```python
from build123d import *

# Parameters (mm, degrees)
F0_R     = 35
F1_DEPTH = 3
F2_R     = 2.75
F3_DEPTH = 3
F4_R     = 26
F5_DEPTH = 3.1
F6_R     = 15
F7_DEPTH = 6.1
F8_SIZE  = 1


with BuildPart() as f1:
    # F0 (on Front) → F1 (new body)
    with BuildSketch(Plane.XZ):
        Circle(F0_R)
    extrude(amount=F1_DEPTH)

    # F2 (on face) → F3 (cut, through all)
    with BuildSketch(Plane.XZ.offset(3)):
        with Locations((30, 0)):
            Circle(F2_R)
        with Locations((0, 30)):
            Circle(F2_R)
        with Locations((-30, 0)):
            Circle(F2_R)
        with Locations((0, -30)):
            Circle(F2_R)
    extrude(amount=-F3_DEPTH, mode=Mode.SUBTRACT)

    # F4 (on face) → F5 (join)
    with BuildSketch(Plane.XZ.offset(3)):
        Circle(F4_R)
    extrude(amount=F5_DEPTH)

    # F6 (on face) → F7 (cut, through all)
    with BuildSketch(Plane.XZ.offset(6.1)):
        Circle(F6_R)
    extrude(amount=-F7_DEPTH, mode=Mode.SUBTRACT)

    # F8
    f8_edges = [f1.edges().sort_by_distance(p)[0] for p in [
        (-26, -6.1, 0),
    ]]
    chamfer(f8_edges, length=F8_SIZE)


solid = f1.part
```
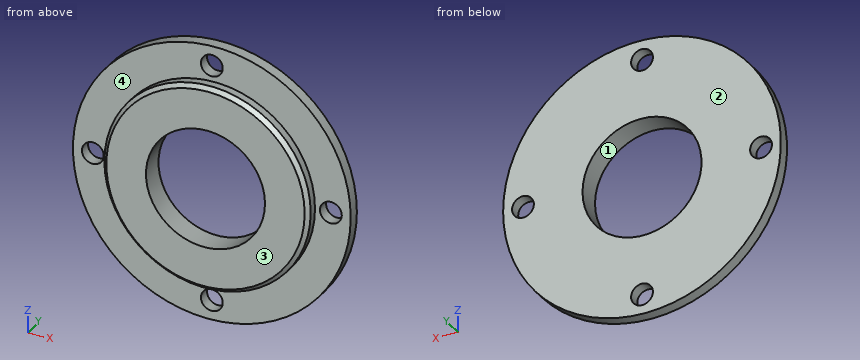
Verification items for the finished model (mm, model axes). Face numbers are marked on the shaded views. A direction names the side the tool comes from. Coordinates: 2 decimals unless noted, no trailing zeros. Loops run counter-clockwise (first coordinate to the right, second up) from the corner with the lowest first, then second, coordinate; pieces in that order, holes last. Notation, with made-up numbers: (69.25, 53.5) -> (107.25, 53.5) arc R13 ccw to (107.25, 63.5) -> close; hole circle Ø6 at (48, 47.25). An arc over 180 degrees is marked (long way). Put each result on its own line as item: value.
1. Thickness scan on line 1 (Z direction, x = 0, y = -2.25); line 2 (Z direction, x = 0, y = -4); line 3 (Z direction, x = -30, y = -1.7). Record the ranges inside material, lowest first.
Result set:
line 1: z = -35 to -32.75, -27.25 to -15, 15 to 27.25, 32.75 to 35
line 2: z = -26 to -15, 15 to 26
line 3: z = -18.03 to -2.75, 2.75 to 18.03
2. Tool access check on the marked faces 3 and 4. Record the directions out of +Z, -Z, +X, -X, +Y, -Y that give a thin tool (end or side, any length) a straight path to the whole face; none if there is none.
Result set:
face 3: +Z, -Z, +X, -X, -Y
face 4: -Y
3. Section check C-C, the plane y = -2. Record the boundary of the cut face in (x, z).
Result set:
outline: circle Ø70 at (0, 0); hole circle Ø5.5 at (-30, 0); hole circle Ø30 at (0, 0); hole circle Ø5.5 at (0, -30); hole circle Ø5.5 at (0, 30); hole circle Ø5.5 at (30, 0)
4. Section check A-A, the plane z = 0. Record the boundary of the cut face in (x, y).
Result set:
outline: (-35, -3) -> (-32.75, -3) -> (-32.75, 0) -> (-35, 0) -> close; (-27.25, -3) -> (-26, -3) -> (-26, -5.1) -> (-25, -6.1) -> (-15, -6.1) -> (-15, 0) -> (-27.25, 0) -> close; (15, -6.1) -> (25, -6.1) -> (26, -5.1) -> (26, -3) -> (27.25, -3) -> (27.25, 0) -> (15, 0) -> close; (32.75, -3) -> (35, -3) -> (35, 0) -> (32.75, 0) -> close
5. Section check B-B, the plane x = 0. Record the boundary of the cut face in (y, z).
Result set:
outline: (-6.1, -25) -> (-5.1, -26) -> (-3, -26) -> (-3, -27.25) -> (0, -27.25) -> (0, -15) -> (-6.1, -15) -> close; (-6.1, 15) -> (0, 15) -> (0, 27.25) -> (-3, 27.25) -> (-3, 26) -> (-5.1, 26) -> (-6.1, 25) -> close; (-3, -35) -> (0, -35) -> (0, -32.75) -> (-3, -32.75) -> close; (-3, 32.75) -> (0, 32.75) -> (0, 35) -> (-3, 35) -> close
6. Gauge pin test, flat ends, axial feed: P1, Ø3.5, axis at x = 30, z = 0, coming from the +Y side; P2, Ø6.5, axis at x = -30, z = 0, coming from the -Y side; P3, Ø6, axis at x = -21.5, z = 18.5, coming from the -Y side; P4, Ø2, axis at x = -4.5, y = -5, coming from the -Z side. Record the tip position at first contact, or that the pin passes through.
Result set:
P1: passes through
P2: stops at y = -3
P3: stops at y = -5.74
P4: stops at z = -25.76
7. Mould release check, pull along X, two halves, no side actions. Record for the marked faces 1 and 2: pulls with the +X half, pulls with the -X half, needs draft (parallel to the pull), parting line crosses it, or undercut.
Result set:
face 1: undercut
face 2: needs draft
8. Section check D-D, the plane x = 30. Record the boundary of the cut face in (y, z), then the cut area to 3 significant figures.
Result set:
outline: (-3, -18.03) -> (0, -18.03) -> (0, -2.75) -> (-3, -2.75) -> close; (-3, 2.75) -> (0, 2.75) -> (0, 18.03) -> (-3, 18.03) -> close
area: 91.7 mm^2
